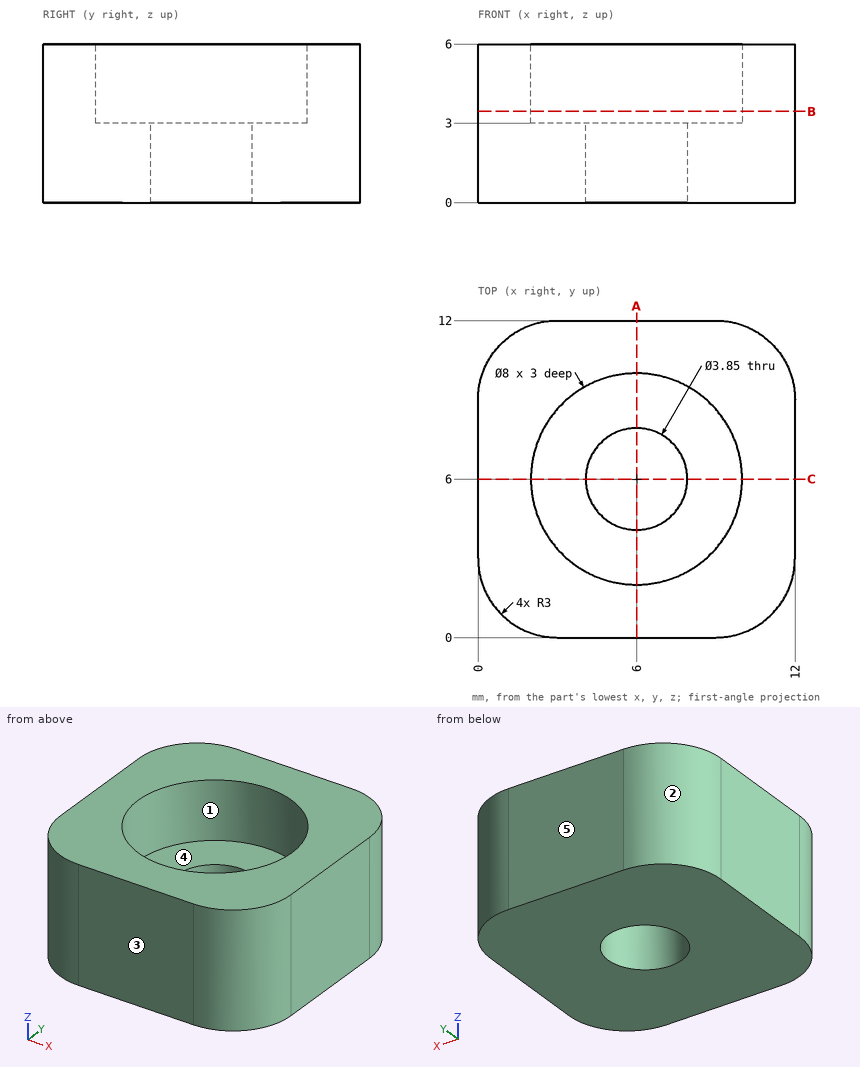
Answer from the drawing. Dimensions are ordinates in mm from the lowest x, y and z of the part. A direction names the side the tool comes from. Give positions to 0.01 mm unless a question says otherwise; leave off trailing zeros. Loops run counter-clockwise (first coordinate to the right, second up) from the corner with the lowest first, then second, coordinate; pieces in that order, holes last. Notation, with made-up numbers: (11, 81.5) -> (39, 81.5) arc R15 ccw to (39, 100.5) -> close; hole circle Ø6 at (63.5, -1). An arc over 180 degrees is marked (long way). One line per question, with ' | ' between items. Start each with the question number.
1) Each of these flat-tipped pins is pushed along its axis until it touches: pin 1 (5 mm diameter, centred on x = 6, y = 6, fed in from -Z); pin 2 (1.5 mm diameter, centred on x = 10, z = 5, fed in from -Y); pin 3 (6.5 mm diameter, centred on x = 6, y = 6, fed in from +Z). Where does it stop, or does it pass through?
2) Determine the mould class of the marked faces 1, 2 and 3 for opening direction X: +X half, -X half, draft (parallel to the pull), parting line (faces both ways), or undercut.
3) For the marked faces 4 and 5, determine the directions among +Z, -Z, +X, -X, +Y, -Y from which every point of the face is accessible in a straight line to the end or side of a thin tool.
4) Straight lines are drawn through the part: L1, parallel to Y at x = 6, z = 5.15; L2, parallel to Y at x = 6, z = 1.65 (3 decimals); L3, parallel to Z at x = 4.75, y = 9.5. For each, find the intervals that lie inside material, in ascending order.
5) Section A-A, the plane x = 6 is taken. Determine the outline of the cut face in (y, z) (3 decimals).
6) Section B-B, the plane z = 3.45 is taken. Determine the outline of the cut face in (x, y).
Resolved:
1) pin 1: z = 0 | pin 2: y = 0.01 | pin 3: z = 3
2) face 1: undercut | face 2: -X half | face 3: draft
3) face 4: +Z | face 5: +Z, -Z, +X, -X, +Y
4) L1: 0 to 2, 10 to 12 | L2: 0 to 4.075, 7.925 to 12 | L3: 0 to 3
5) outline: (0, 0) -> (4.075, 0) -> (4.075, 3) -> (2, 3) -> (2, 6) -> (0, 6) -> close; (7.925, 0) -> (12, 0) -> (12, 6) -> (10, 6) -> (10, 3) -> (7.925, 3) -> close
6) outline: (0, 3) arc R3 ccw to (3, 0) -> (9, 0) arc R3 ccw to (12, 3) -> (12, 9) arc R3 ccw to (9, 12) -> (3, 12) arc R3 ccw to (0, 9) -> close; hole circle Ø8 at (6, 6)
